```python
from build123d import *

# Parameters (mm, degrees)
BASEPLATE_OUTLINE_R = 2.1
BASEPLATE_DEPTH     = 2.8
CUT_EXTRUDE1_REACH  = 115.438
SKETCH3_R           = 14
SKETCH3_R_2         = 1.6
SKETCH3_W           = 21
SKETCH3_H           = 3.7
SKETCH3_W_2         = 32
SKETCH3_H_2         = 2.2
SKETCH3_W_3         = 8.1
SKETCH3_H_3         = 57


# Read off the part's stored shape, not the designer's step: BasePlate
with BuildPart() as part:
    # BasePlate outline → BasePlate (new body)
    with BuildSketch(Plane(origin=(0, 0, 0), x_dir=(1, 0, 0), z_dir=(0, 1, 0))):
        with BuildLine():
            Line((43.502626614, -5.852332608), (48.792614178, -5.852332608))
            ThreePointArc((48.792614178, -5.852332608), (49.082078508, -5.760021707), (49.264659986, -5.517174213))
            Line((49.264659986, -5.517174213), (50.078201202, -3.187491002))
            ThreePointArc((50.078201202, -3.187491002), (50.26078268, -2.944643509), (50.55024701, -2.852332608))
            Line((50.55024701, -2.852332608), (58.116695703, -2.852332608))
            ThreePointArc((58.116695703, -2.852332608), (58.484685739, -3.013831008), (58.614956567, -3.393999275))
            ThreePointArc((58.614956567, -3.393999275), (64.799237397, -7.61016844), (65.229166667, -0.137781095))
            ThreePointArc((65.229166667, -0.137781095), (65.061014427, 0.043158816), (65, 0.282515593))
            Line((65, 0.282515593), (65, 83.012819192))
            ThreePointArc((65, 83.012819192), (65.061014427, 83.252175969), (65.229166667, 83.433115879))
            ThreePointArc((65.229166667, 83.433115879), (65.940559159, 90.088226551), (59.285448487, 89.376834059))
            ThreePointArc((59.285448487, 89.376834059), (59.104508577, 89.208681819), (58.8651518, 89.147667392))
            Line((58.8651518, 89.147667392), (6.1348482, 89.147667392))
            ThreePointArc((6.1348482, 89.147667392), (5.895491423, 89.208681819), (5.714551513, 89.376834059))
            ThreePointArc((5.714551513, 89.376834059), (-0.940559159, 90.088226551), (-0.229166667, 83.433115879))
            ThreePointArc((-0.229166667, 83.433115879), (-0.061014427, 83.252175969), (0, 83.012819192))
            Line((0, 83.012819192), (0, 0.282515593))
            ThreePointArc((0, 0.282515593), (-0.061014427, 0.043158816), (-0.229166667, -0.137781095))
            ThreePointArc((-0.229166667, -0.137781095), (0.200762603, -7.61016844), (6.385043433, -3.393999275))
            ThreePointArc((6.385043433, -3.393999275), (6.515314261, -3.013831008), (6.883304297, -2.852332608))
            Line((6.883304297, -2.852332608), (14.44975299, -2.852332608))
            ThreePointArc((14.44975299, -2.852332608), (14.73921732, -2.944643509), (14.921798798, -3.187491002))
            Line((14.921798798, -3.187491002), (15.735340014, -5.517174213))
            ThreePointArc((15.735340014, -5.517174213), (15.917921492, -5.760021707), (16.207385822, -5.852332608))
            Line((16.207385822, -5.852332608), (21.497373386, -5.852332608))
            ThreePointArc((21.497373386, -5.852332608), (21.786837716, -5.760021707), (21.969419194, -5.517174213))
            Line((21.969419194, -5.517174213), (22.78296041, -3.187491002))
            ThreePointArc((22.78296041, -3.187491002), (22.965541888, -2.944643509), (23.255006218, -2.852332608))
            Line((23.255006218, -2.852332608), (41.744993782, -2.852332608))
            ThreePointArc((41.744993782, -2.852332608), (42.034458112, -2.944643509), (42.21703959, -3.187491002))
            Line((42.21703959, -3.187491002), (43.030580806, -5.517174213))
            ThreePointArc((43.030580806, -5.517174213), (43.213162284, -5.760021707), (43.502626614, -5.852332608))
        make_face()
        with Locations((2.1, -3.752332608)):
            Circle(BASEPLATE_OUTLINE_R, mode=Mode.SUBTRACT)
        with Locations((62.9, -3.752332608)):
            Circle(BASEPLATE_OUTLINE_R, mode=Mode.SUBTRACT)
        with Locations((2.1, 87.047667392)):
            Circle(BASEPLATE_OUTLINE_R, mode=Mode.SUBTRACT)
        with Locations((62.9, 87.047667392)):
            Circle(BASEPLATE_OUTLINE_R, mode=Mode.SUBTRACT)
    extrude(amount=BASEPLATE_DEPTH)

    # Sketch3 → Cut-Extrude1 (cut, up to next)
    with BuildSketch(Plane(origin=(0, 2.8, 0), x_dir=(1, 0, 0), z_dir=(0, 1, 0)), mode=Mode.PRIVATE) as cut_extrude1_sk1:
        with Locations(Location((29.45, 21.897667392, 0), (0, 0, 270))):
            Circle(SKETCH3_R)
    cut_extrude1_tool1 = extrude(cut_extrude1_sk1.sketch, amount=-CUT_EXTRUDE1_REACH, mode=Mode.PRIVATE) & part.part
    # Sketch3 → Cut-Extrude1 (cut, up to next)
    with BuildSketch(Plane(origin=(0, 2.8, 0), x_dir=(1, 0, 0), z_dir=(0, 1, 0)), mode=Mode.PRIVATE) as cut_extrude1_sk2:
        with Locations(Location((41.45, 33.897667392, 0), (0, 0, 270))):
            Circle(SKETCH3_R_2)
    cut_extrude1_tool2 = extrude(cut_extrude1_sk2.sketch, amount=-CUT_EXTRUDE1_REACH, mode=Mode.PRIVATE) & part.part
    # Sketch3 → Cut-Extrude1 (cut, up to next)
    with BuildSketch(Plane(origin=(0, 2.8, 0), x_dir=(1, 0, 0), z_dir=(0, 1, 0)), mode=Mode.PRIVATE) as cut_extrude1_sk3:
        with Locations(Location((41.45, 9.897667392, 0), (0, 0, 270))):
            Circle(SKETCH3_R_2)
    cut_extrude1_tool3 = extrude(cut_extrude1_sk3.sketch, amount=-CUT_EXTRUDE1_REACH, mode=Mode.PRIVATE) & part.part
    # Sketch3 → Cut-Extrude1 (cut, up to next)
    with BuildSketch(Plane(origin=(0, 2.8, 0), x_dir=(1, 0, 0), z_dir=(0, 1, 0)), mode=Mode.PRIVATE) as cut_extrude1_sk4:
        with Locations(Location((17.45, 9.897667392, 0), (0, 0, 270))):
            Circle(SKETCH3_R_2)
    cut_extrude1_tool4 = extrude(cut_extrude1_sk4.sketch, amount=-CUT_EXTRUDE1_REACH, mode=Mode.PRIVATE) & part.part
    # Sketch3 → Cut-Extrude1 (cut, up to next)
    with BuildSketch(Plane(origin=(0, 2.8, 0), x_dir=(1, 0, 0), z_dir=(0, 1, 0)), mode=Mode.PRIVATE) as cut_extrude1_sk5:
        with Locations(Location((17.45, 33.897667392, 0), (0, 0, 270))):
            Circle(SKETCH3_R_2)
    cut_extrude1_tool5 = extrude(cut_extrude1_sk5.sketch, amount=-CUT_EXTRUDE1_REACH, mode=Mode.PRIVATE) & part.part
    # Sketch3 → Cut-Extrude1 (cut, up to next)
    with BuildSketch(Plane(origin=(0, 2.8, 0), x_dir=(1, 0, 0), z_dir=(0, 1, 0)), mode=Mode.PRIVATE) as cut_extrude1_sk6:
        with Locations((32.5, 2.897667392)):
            Rectangle(SKETCH3_W, SKETCH3_H)
    cut_extrude1_tool6 = extrude(cut_extrude1_sk6.sketch, amount=-CUT_EXTRUDE1_REACH, mode=Mode.PRIVATE) & part.part
    # Sketch3 → Cut-Extrude1 (cut, up to next)
    with BuildSketch(Plane(origin=(0, 2.8, 0), x_dir=(1, 0, 0), z_dir=(0, 1, 0)), mode=Mode.PRIVATE) as cut_extrude1_sk7:
        with Locations((50.5, 44.897667392)):
            Rectangle(SKETCH3_W, SKETCH3_H)
    cut_extrude1_tool7 = extrude(cut_extrude1_sk7.sketch, amount=-CUT_EXTRUDE1_REACH, mode=Mode.PRIVATE) & part.part
    # Sketch3 → Cut-Extrude1 (cut, up to next)
    with BuildSketch(Plane(origin=(0, 2.8, 0), x_dir=(1, 0, 0), z_dir=(0, 1, 0)), mode=Mode.PRIVATE) as cut_extrude1_sk8:
        with Locations((22.55, 86.247667392)):
            Rectangle(SKETCH3_W_2, SKETCH3_H_2)
    cut_extrude1_tool8 = extrude(cut_extrude1_sk8.sketch, amount=-CUT_EXTRUDE1_REACH, mode=Mode.PRIVATE) & part.part
    # Sketch3 → Cut-Extrude1 (cut, up to next)
    with BuildSketch(Plane(origin=(0, 2.8, 0), x_dir=(1, 0, 0), z_dir=(0, 1, 0)), mode=Mode.PRIVATE) as cut_extrude1_sk9:
        with Locations((8.85, 31.547667392)):
            Rectangle(SKETCH3_W_3, SKETCH3_H_3)
    cut_extrude1_tool9 = extrude(cut_extrude1_sk9.sketch, amount=-CUT_EXTRUDE1_REACH, mode=Mode.PRIVATE) & part.part
    add(cut_extrude1_tool1.solids().sort_by_distance((29.45, 2.8, -21.897667))[0], mode=Mode.SUBTRACT)
    add(cut_extrude1_tool2.solids().sort_by_distance((41.45, 2.8, -33.897667))[0], mode=Mode.SUBTRACT)
    add(cut_extrude1_tool3.solids().sort_by_distance((41.45, 2.8, -9.897667))[0], mode=Mode.SUBTRACT)
    add(cut_extrude1_tool4.solids().sort_by_distance((17.45, 2.8, -9.897667))[0], mode=Mode.SUBTRACT)
    add(cut_extrude1_tool5.solids().sort_by_distance((17.45, 2.8, -33.897667))[0], mode=Mode.SUBTRACT)
    add(cut_extrude1_tool6.solids().sort_by_distance((32.5, 2.8, -2.897667))[0], mode=Mode.SUBTRACT)
    add(cut_extrude1_tool7.solids().sort_by_distance((50.5, 2.8, -44.897667))[0], mode=Mode.SUBTRACT)
    add(cut_extrude1_tool8.solids().sort_by_distance((22.55, 2.8, -86.247667))[0], mode=Mode.SUBTRACT)
    add(cut_extrude1_tool9.solids().sort_by_distance((8.85, 2.8, -31.547667))[0], mode=Mode.SUBTRACT)


solid = part.part
```
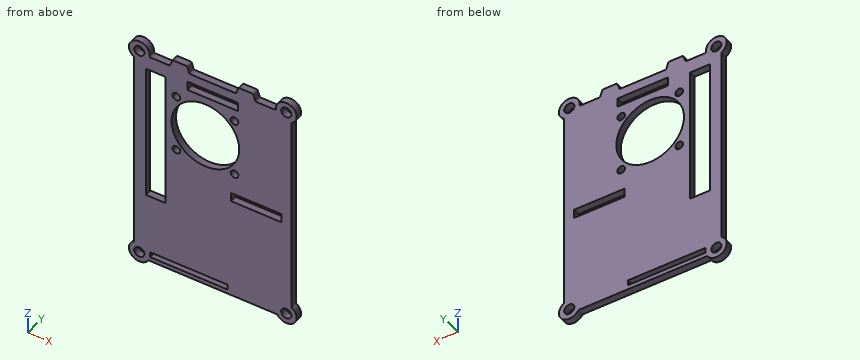
Geometry check sheet. Reference: the model listing, model coordinates, mm. Give positions to 0.01 mm unless a question says otherwise; leave off trailing zeros. Write each loop counter-clockwise with the first axis right and the second up, starting at its lowest first coordinate (ties: lowest second). Pieces come first, ordered by that corner, then holes. Notation, with made-up numbers: (-33.5, -9.5) -> (8.5, -9.5) arc R32 ccw to (8.5, 29.5) -> close; hole circle Ø1 at (75, 9). An arc over 180 degrees is marked (long way). Use one line per item in the form item = value.
Item 1: Sectioned sample at A-A on z = -52. Enter the section's corners in (x, y), plus the area to 3 significant figures.
Results list:
outline = (0, 0) -> (4.8, 0) -> (4.8, 2.8) -> (0, 2.8) -> close; (12.9, 0) -> (65, 0) -> (65, 2.8) -> (12.9, 2.8) -> close
area = 159 mm2
Item 2: Depth check by flat-ended pin: pin 1 Ø0.8 at (x, y) = (46.5, 2) entering from +Z; pin 2 Ø0.8 at (y, z) = (1.5, -44.5) entering from -X; pin 3 Ø1.4 at (y, z) = (1, -23.5) entering from +X. Enter the tip coordinate at first touch or a pass-through.
Results list:
pin_1 = 5.85
pin_2 = 0
pin_3 = 65
Item 3: Sectioned sample at D-D on x = 53.5. Enter the section's corners in (y, z).
Results list:
outline = (0, -89.15) -> (2.8, -89.15) -> (2.8, -46.75) -> (0, -46.75) -> close; (0, -43.05) -> (2.8, -43.05) -> (2.8, 2.85) -> (0, 2.85) -> close
Item 4: Scan lines: line 1 (X direction, y = 2.65, z = -4.5); line 2 (Z direction, x = 2.1, y = 0.75); line 3 (X direction, y = 1.25, z = -22). Record each from-to range of solid material in increasing order.
Results list:
line_1 = 0 to 4.8, 12.9 to 22, 43 to 65
line_2 = -91.35 to -89.15, -84.95 to 1.65, 5.85 to 8.05
line_3 = 0 to 4.8, 12.9 to 15.45, 43.45 to 65
Item 5: Sectioned sample at B-B on x = 2.1. Enter the section's corners in (y, z), plus the area to 3 significant figures.
Results list:
outline = (0, -91.35) -> (2.8, -91.35) -> (2.8, -89.15) -> (0, -89.15) -> close; (0, -84.95) -> (2.8, -84.95) -> (2.8, 1.65) -> (0, 1.65) -> close; (0, 5.85) -> (2.8, 5.85) -> (2.8, 8.05) -> (0, 8.05) -> close
area = 255 mm2
Item 6: Sectioned sample at C-C on x = 29.45. Enter the section's corners in (y, z).
Results list:
outline = (0, -89.15) -> (2.8, -89.15) -> (2.8, -87.35) -> (0, -87.35) -> close; (0, -85.15) -> (2.8, -85.15) -> (2.8, -35.9) -> (0, -35.9) -> close; (0, -7.9) -> (2.8, -7.9) -> (2.8, -4.75) -> (0, -4.75) -> close; (0, -1.05) -> (2.8, -1.05) -> (2.8, 2.85) -> (0, 2.85) -> close
